Autodesk Inventor part; units mm, degrees
ref_plane "YZ Plane" through (0, 0, 0) normal (1, 0, 0) x (0, 1, 0)
ref_plane "XZ Plane" through (0, 0, 0) normal (0, 1, 0) x (-1, 0, 0)
ref_plane "XY Plane" through (0, 0, 0) normal (0, 0, 1) x (1, 0, 0)
sketch "Sketch1" plane through (0, 0, 0) normal (0, 0, 1) x (1, 0, 0)
  line L0 (-8.5, 42.6) -> (-6.1, 42.6)
  line L1 (-6.1, 36.1) -> (-8.5, 36.1)
  line L2 (-6.1, 36.1) -> (-6.1, 42.6)
  line L3 (-8.5, 37.35) -> (-8.5, 36.1)
  line L4 (-8.5, 41.35) -> (-8.5, 42.6)
  line L5 (-8.5, 37.35) -> (-9.2058, 37.35)
  line L6 (-8.5, 41.35) -> (-9.2058, 41.35)
  line L7 (-9.9, 42.36) -> (-9.2058, 41.35)
  line L8 (-9.9, 36.34) -> (-9.2058, 37.35)
  line L9 (-9.9, 36.34) -> (-13.4, 36.34)
  line L10 (-9.9, 42.36) -> (-13.4, 42.36)
  line L11 (-13.4, 42.36) -> (-13.4, 36.34)
  point P0 (-8.5, 41.975)
  point P1 (-6.1, 39.35)
  dimension "d27" = 6.5
  dimension "d28" = 2.4
  dimension "d29" = 2.4
  dimension "d35" = 111
  dimension "d36" = 4
  dimension "d37" = 6.02
  dimension "d38" = 0.7058
  dimension "d39" = 0.7058
  dimension "d43" = 3.01
  dimension "d44" = 2
  dimension "d63" = 3.5
  dimension "d64" = 3.5
extrude "Extrusion1" add sketch "Sketch1" against normal blind 1025.4
ref_plane "Plano de trabajo3" through (0, 0, -512.7) normal (0, 0, 1) x (1, 0, 0)
sketch "Boceto2" plane through (-6.1, 36.1, 0) normal (1, 0, 0) x (0, 0, -1)
  line L0 (0, 0) -> (6.5, 6.5)
  line L1 (0, 6.5) -> (1025.4, 6.5)
  line L2 (6.5, 6.5) -> (0, 6.5)
  line L3 (6.5, 6.5) -> (0, 6.5)
  line L4 (0, 6.5) -> (0, 0)
  point P0 (0, -36.1)
  dimension "d65" = 45
extrude "Extrusión3" cut sketch "Boceto2" against normal through all
mirror "Simetría3" about plane through (0, 0, -512.7) normal (0, 0, 1) of "Extrusión3"
properties part number "SP40-10 JUNTA INT 1026.2 mm" material "Rubber"
Part model, mm, in its own coordinate system. Round coordinates to 2 decimals unless told otherwise and drop trailing zeros. Write each loop counter-clockwise with the first axis right and the second up, starting at its lowest first coordinate (ties: lowest second). Pieces come first, ordered by that corner, then holes. Notation, with made-up numbers: (-19, 50) -> (19, 50) arc R27 ccw to (19, 70) -> close; hole circle Ø1 at (-16.75, -18.75). An arc over 180 degrees is marked (long way). Return JSON: item names as keys, results as strings. Group by question number.
Q1. Pin check, flat tips, straight feed: pin 1 (1 mm diameter, centred on x = -12, z = -530, fed in from +Y); pin 2 (3 mm diameter, centred on x = -12.5, z = -745, fed in from -Y); pin 3 (0.8 mm diameter, centred on x = -9, z = -283, fed in from -Y). Stop position of each tip, or through.
Q2. Probe L1, parallel to Z at x = -9, y = 41.25; L2, parallel to Y at x = -10.5, z = -889; L3, parallel to X at y = 42.25, z = -59. List the from-to ranges inside material, lowest first. Write a range as [from, to].
Q3. Saw through at B-B on x = -11.75. Write the cut outline in (y, z).
Q4. Saw through at A-A on z = -379.5. Write the cut outline in (x, y), plus the area to 3 significant figures.
Answer:
{
 "1": {"pin 1": "y = 42.36", "pin 2": "y = 36.34", "pin 3": "y = 37.07"},
 "2": {"L1": "[-1020.25, -5.15]", "L2": "[36.34, 42.36]", "L3": "[-13.4, -9.82], [-8.5, -6.1]"},
 "3": {"outline": "(36.34, -1025.16) -> (42.36, -1019.14) -> (42.36, -6.26) -> (36.34, -0.24) -> close"},
 "4": {"outline": "(-13.4, 36.34) -> (-9.9, 36.34) -> (-9.21, 37.35) -> (-8.5, 37.35) -> (-8.5, 36.1) -> (-6.1, 36.1) -> (-6.1, 42.6) -> (-8.5, 42.6) -> (-8.5, 41.35) -> (-9.21, 41.35) -> (-9.9, 42.36) -> (-13.4, 42.36) -> close", "area": "43.0 mm2"}
}
